CAD build for the part. Positions are in the model's coordinates, mm. A direction names the side the tool comes from. Coordinates: 2 decimals unless noted, no trailing zeros. Write each loop counter-clockwise with the first axis right and the second up, starting at its lowest first coordinate (ties: lowest second). Pieces come first, ordered by that corner, then holes.
```python
from build123d import *

# Parameters (mm, degrees)
BOSS_EXTRUDE1_DEPTH = 0.635
BOSS_EXTRUDE2_REACH = 31.451
SKETCH2_R           = 1.42875
SKETCH3_W           = 5.08
SKETCH3_H           = 7
CUT_EXTRUDE1_DEPTH  = 40
SKETCH4_R           = 0.79375
CUT_EXTRUDE2_DEPTH  = 40
FILLET1_R           = 2.5


with BuildPart() as part:
    # Sketch1 → Boss-Extrude1 (new body)
    with BuildSketch(Plane(origin=(0, 0, 0), x_dir=(1, 0, 0), z_dir=(0, 1, 0))):
        Polygon((-6.689871172, 14.89260144), (-11.769871172, 14.89260144), (-11.769871172, 0.76385144), (13.630128828, 0.76385144), (13.630128828, 14.89260144), (8.550128828, 14.89260144), (8.550128828, 7.89260144), (3.470128828, 7.89260144), (3.470128828, 14.89260144), (-1.609871172, 14.89260144), (-1.609871172, 7.89260144), (-6.689871172, 7.89260144), align=None)
    extrude(amount=BOSS_EXTRUDE1_DEPTH)

    # Boss-Extrude2: up to this face of the body (flat: up to its plane)
    boss_extrude2_end = Plane(part.part.faces().sort_by_distance((-11.769871172, 0.3175, -7.82822644))[0])
    # Sketch2 → Boss-Extrude2 (add, up to the picked face)
    with BuildSketch(Plane(origin=(13.630128828, 0, 0), x_dir=(0, 0, -1), z_dir=(1, 0, 0)), mode=Mode.PRIVATE) as boss_extrude2_sk1:
        with Locations(Location((13.46385144, -0.79375, 0), (0, 0, 33.748988596))):
            Circle(SKETCH2_R)
    boss_extrude2_tool1 = split(extrude(boss_extrude2_sk1.sketch, amount=-BOSS_EXTRUDE2_REACH, mode=Mode.PRIVATE), bisect_by=boss_extrude2_end, keep=Keep.BOTH, mode=Mode.PRIVATE)
    add(boss_extrude2_tool1.solids().sort_by(Axis((13.630129, -0.79375, -13.463851), (-1, 0, 0)))[0])

    # Sketch3 → Cut-Extrude1 (cut)
    with BuildSketch(Plane(origin=(0, 0.635, 0), x_dir=(1, 0, 0), z_dir=(0, 1, 0))):
        with Locations((-4.149871172, 11.39260144)):
            Rectangle(SKETCH3_W, SKETCH3_H)
        with Locations((6.010128828, 11.39260144)):
            Rectangle(SKETCH3_W, SKETCH3_H)
    extrude(amount=-CUT_EXTRUDE1_DEPTH, mode=Mode.SUBTRACT)

    # Sketch4 → Cut-Extrude2 (cut)
    with BuildSketch(Plane(origin=(13.630128828, 0, 0), x_dir=(0, 0, -1), z_dir=(1, 0, 0))):
        with Locations((13.46385144, -0.79375)):
            Circle(SKETCH4_R)
    extrude(amount=-CUT_EXTRUDE2_DEPTH, mode=Mode.SUBTRACT)

    # Fillet1
    # the kernel refuses this fillet: 2.5 mm, written as the material it takes off along each edge
    with BuildSketch(Plane(origin=(-2.527709024, 0.635, -14.89260144), x_dir=(0, 0, 1), z_dir=(-1, 0, 0)), Plane(origin=(7.632290976, 0.635, -14.89260144), x_dir=(0, 0, 1), z_dir=(-1, 0, 0))) as fillet1_piece_1:
        with BuildLine():
            CenterArc((1.664864859, -2.5), FILLET1_R, 90, 41.754936598)
            Line((0, -0.635), (-0.033297297, -0.5977))
            ThreePointArc((-0.033297297, -0.5977), (-0.05, -0.3175), (-0.05, 0))
            Line((-0.05, 0), (0, 0.05))
            Line((0, 0.05), (1.664864859, 0.05))
            Line((1.664864859, 0.05), (1.664864859, 0))
        make_face()
    extrude(amount=13.404324297, mode=Mode.SUBTRACT)
    with BuildSketch(Plane(origin=(17.792290976, 0.635, -14.89260144), x_dir=(0, -1, 0), z_dir=(-1, 0, 0))) as fillet1_piece_2:
        with BuildLine():
            CenterArc((2.5, 1.664864859), FILLET1_R, 180, 41.754936598)
            Line((0, 1.664864859), (-0.05, 1.664864859))
            Line((-0.05, 1.664864859), (-0.05, 0))
            Line((-0.05, 0), (0, -0.05))
            ThreePointArc((0, -0.05), (0.3175, -0.05), (0.5977, -0.033297297))
            Line((0.5977, -0.033297297), (0.635, 0))
        make_face()
    extrude(amount=13.404324297, mode=Mode.SUBTRACT)


solid = part.part
```
Item 1: Saw through at D-D, the plane x = -5. Write the cut outline in (y, z) (3 decimals), and give its area (3 significant figures).
Item 2: Saw through at B-B, the plane y = -0.5. Write the cut outline in (x, z).
Item 3: Two-plate mould, pull along Y, no slides. Class faces 3 (the flat face through (-1.61, -0.5, -12.22)), 4 (the cylindrical face through (-9.194, -1.098, -14.197)), 5 (the cylindrical face through (11.126, 0.475, -14.107)): +Y half, -Y half, draft (parallel to the pull), parting line (faces both ways), or undercut.
Item 4: Which spindle directions (+Z, -Z, +X, -X, +Y, -Y) get a long thin tool onto all of the face, cutting with end or side? Do faces 1 (the cylindrical face through (-9.194, 0.475, -14.107)), 2 (the flat face through (-6.69, 0.1, -12.9)). Say none if no direction does.
Item 5: Wall check: line 1 along X through (y, z) = (-1.55, -14); line 2 along Z through (x, y) = (-7.25, -0.8); line 3 along Z through (x, y) = (7, 0.05). Give the ranges that are in metal, low to high.
Item 6: Saw through at C-C, the plane z = -7. Write the cut outline in (x, y) (3 decimals), and give its area (3 significant figures).
Item 7: Flat gauge pin, fed straight in: pin 1 Ø0.7 at (x, y) = (6.5, 0.5) entering from -Z. Where does the tip first touch, or does it go through?
Working result:
1. outline: (0, -7.893) - (0.635, -7.893) - (0.635, -0.764) - (0, -0.764) - close
1. area: 4.53 mm2
2. outline: (-11.77, -14.86) - (-6.69, -14.86) - (-6.69, -14.2) - (-11.77, -14.2) - close; (-11.77, -12.73) - (-6.69, -12.73) - (-6.69, -12.07) - (-11.77, -12.07) - close; (-1.61, -14.86) - (3.47, -14.86) - (3.47, -14.2) - (-1.61, -14.2) - close; (-1.61, -12.73) - (3.47, -12.73) - (3.47, -12.07) - (-1.61, -12.07) - close; (8.55, -14.86) - (13.63, -14.86) - (13.63, -14.2) - (8.55, -14.2) - close; (8.55, -12.73) - (13.63, -12.73) - (13.63, -12.07) - (8.55, -12.07) - close
3. face 3: draft
3. face 4: undercut
3. face 5: +Y half
4. face 1: -Z, +X, -X, +Y
4. face 2: -Z, +Y, -Y
5. line 1: x = -11.77 to -6.69, -1.61 to 3.47, 8.55 to 13.63
5. line 2: z = -14.89 to -14.26, -12.67 to -12.04
5. line 3: z = -7.89 to -0.76
6. outline: (-11.77, 0) - (13.63, 0) - (13.63, 0.635) - (-11.77, 0.635) - close
6. area: 16.1 mm2
7. pin 1: stops at z = -7.89
